The model under review builds one solid part; all positions refer to its coordinate system, in mm. Coordinates: 2 decimals unless noted, no trailing zeros. Write each loop counter-clockwise with the first axis right and the second up, starting at its lowest first coordinate (ties: lowest second). Pieces come first, ordered by that corner, then holes. Notation, with made-up numbers: (75, -8) - (89, -8) arc R14 cw to (89, 19) - close; hole circle Ø6 at (78.5, -20.5). An arc over 180 degrees is marked (long way). Put each result on its own line as item: value. Start each with the question number.
Item 1: Consider section A-A on z = 1774.5. Give the boundary of the cut face in (x, y).
Item 2: For pin 1 (5 mm diameter, centred on y = 0, z = 2375, fed in from -X), flat-tipped, find the tip position at first contact; note if it passes through.
Item 3: To check wall thickness, follow L1, parallel to Z at x = -19, y = 0; L2, parallel to Y at x = -11, z = 1339. State the ranges of each line that lie inside material, in increasing order. Write a range as [from, to].
Autodesk Inventor part; units mm, degrees
ref_plane "Start Plane" through (0, 0, 0) normal (0, 0, 1) x (1, 0, 0)
ref_plane "End Plane" through (0, 0, 2500) normal (0, 0, 1) x (1, 0, 0)
ref_plane "YZ Plane" through (0, 0, 0) normal (1, 0, 0) x (0, 1, 0)
ref_plane "Start Plane" through (0, 0, 0) normal (0, 0, 1) x (1, 0, 0)
ref_plane "End Plane" through (0, 0, 2500) normal (0, 0, 1) x (1, 0, 0)
sketch "Sketch" plane through (0, 0, 0) normal (0, 0, 1) x (1, 0, 0)
  line L0 (-20, -16) -> (-20, 16)
  line L1 (-16, 20) -> (16, 20)
  line L2 (20, 16) -> (20, -16)
  line L3 (16, -20) -> (-16, -20)
  arc A0 (-20, -16) -> (-16, -20) centre (-16, -16) ccw
  arc A1 (20, 16) -> (16, 20) centre (16, 16) ccw
  arc A2 (-16, 20) -> (-20, 16) centre (-16, 16) ccw
  arc A3 (16, -20) -> (20, -16) centre (16, -16) ccw
  arc A4 (-16, 18) -> (-18, 16) centre (-16, 16) ccw
  line L4 (-16, 18) -> (16, 18)
  arc A5 (18, 16) -> (16, 18) centre (16, 16) ccw
  line L5 (18, 16) -> (18, -16)
  arc A6 (16, -18) -> (18, -16) centre (16, -16) ccw
  line L6 (16, -18) -> (-16, -18)
  arc A7 (-18, -16) -> (-16, -18) centre (-16, -16) ccw
  line L7 (-18, -16) -> (-18, 16)
  line L8 (0, 29.1598) -> (0, -29.1598) construction
  line L9 (-29.1598, 0) -> (29.1598, 0) construction
  dimension "d7" = 4
  dimension "d9" = 40
  dimension "d11" = 40
  dimension "d12" = 2
  dimension "d15" = 20
  dimension "d16" = 20
extrude "Body" add sketch "Sketch" along normal up to surface (2500 mm away) from surface at 0
sketch "Sketch3" plane through (0, 0, 0) normal (0, 0, 1) x (1, 0, 0)
  line L0 (0, 0) -> (10, 0)
ref_plane "Work Plane3" through (0, 0, 0) normal (0, -1, 0) x (1, 0, 0)
sketch "Sketch5" plane through (0, 0, 0) normal (1, 0, 0) x (0, 1, 0)
  circle A0 centre (0, 2325) radius 2.75
  circle A1 centre (0, 2375) radius 2.75
  circle A2 centre (0, 2475) radius 2.75
  circle A3 centre (0, 2425) radius 2.75
  line L0 (16, 2500) -> (-16, 2500)
  point P0 (0, 0)
  point P1 (0, 2500)
  dimension "d19" = 5.5
  dimension "d21" = 50
  dimension "d22" = 50
  dimension "d23" = 50
  dimension "d25" = 25
extrude "Extrusion2" cut sketch "Sketch5" along normal through all both and the other way through all
pattern_circular "Circular Pattern1" count 2 over 90 about axis through (0, 0, -10) along (0, 0, 1) of "Extrusion2"
sketch "Sketch4" plane through (0, 0, 0) normal (0, -1, 0) x (1, 0, 0)
  line L0 (-2, 0) -> (12, 0)
  line L1 (-2, 2500) -> (12, 2500)
  dimension "d18" = 2500
equation "\"d7\" = G_IR"
equation "\"d9\" = G_W"
equation "\"d11\" = G_H"
equation "\"d12\" = G_T"
equation "\"d15\" = 0.5 * d9"
equation "\"d16\" = 0.5 * d11"
equation "\"d3\" = G_L"
equation "\"d22\" = d21"
equation "\"d23\" = d21"
equation "\"d25\" = 0.5 * d21"
equation "\"G_W\" = 40"
equation "\"G_H\" = 40"
equation "\"G_T\" = 2"
equation "\"G_IR\" = 4"
equation "\"G_L\" = d18"
equation "\"G_OFFSET_START\" = 0"
equation "\"G_OFFSET_END\" = 0"
properties part number "ISO 10799-2 - 40x40x2 - 2500" material "Stainless Steel"
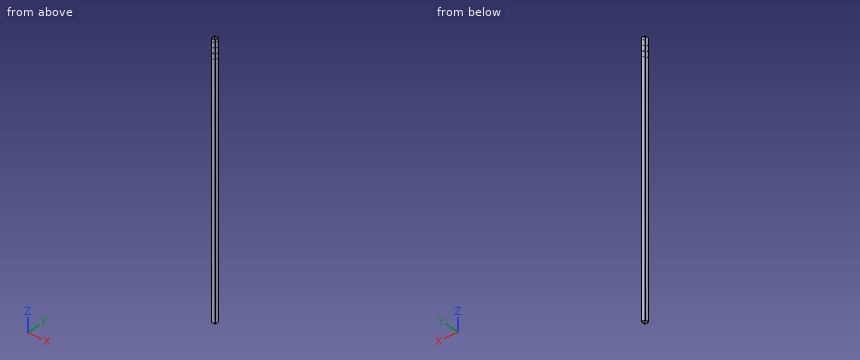
Report:
1. outline: (-20, -16) arc R4 ccw to (-16, -20) - (16, -20) arc R4 ccw to (20, -16) - (20, 16) arc R4 ccw to (16, 20) - (-16, 20) arc R4 ccw to (-20, 16) - close; hole (-18, -16) arc R2 ccw to (-16, -18) - (16, -18) arc R2 ccw to (18, -16) - (18, 16) arc R2 ccw to (16, 18) - (-16, 18) arc R2 ccw to (-18, 16) - close
2. pin 1: through
3. L1: [0, 2322.25], [2327.75, 2372.25], [2377.75, 2422.25], [2427.75, 2472.25], [2477.75, 2500]
3. L2: [-20, -18], [18, 20]
